Read the model definition and answer for the solid it produces. Units are mm, in the model's axes. Face numbers are marked on the shaded views. A direction names the side the tool comes from. Round coordinates to 2 decimals unless told otherwise and drop trailing zeros. Order: outer loops, then holes, each group sorted by start corner. A loop starts at its lowest first (then second) coordinate and runs counter-clockwise, first axis right, second up.
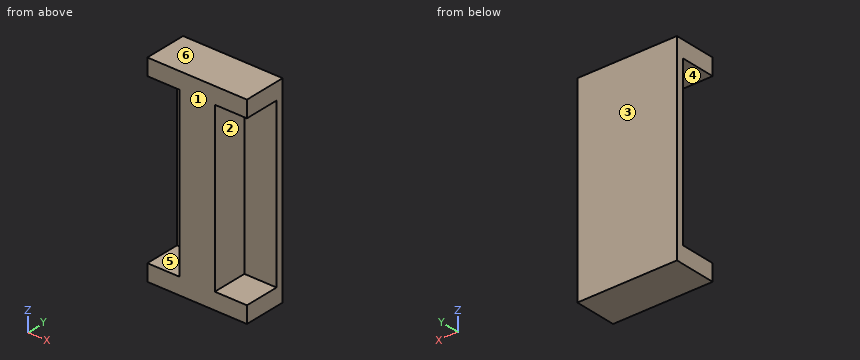
from build123d import *

# Parameters (mm, degrees)
F0_W     = 609.6
F0_H     = 1219.2
F1_DEPTH = 44.45
F2_W     = 609.6
F2_H     = 101.6
F3_DEPTH = 215.9
F4_W     = 215.9
F4_H     = 1016
F5_DEPTH = 260.35


with BuildPart() as f1:
    # F0 (on Front) → F1 (new body)
    with BuildSketch(Plane.XZ):
        Rectangle(F0_W, F0_H)
    extrude(amount=F1_DEPTH)

    # F2 (on face) → F3 (join)
    with BuildSketch(Plane.XZ.offset(44.45)):
        with Locations((0, 558.8)):
            Rectangle(F2_W, F2_H)
        with Locations((0, -558.8)):
            Rectangle(F2_W, F2_H)
    extrude(amount=F3_DEPTH)

    # F4 (on Front) → F5 (join)
    with BuildSketch(Plane.XZ):
        Rectangle(F4_W, F4_H)
    extrude(amount=F5_DEPTH)


solid = f1.part
Q1. For the marked faces 1 and 2, determine the directions among +Z, -Z, +X, -X, +Y, -Y from which every point of the face is accessible in a straight line to the end or side of a thin tool.
Outcome:
face 1: +Z, -Z, +X, -X, -Y
face 2: +X, -Y
Q2. A cutting plane is placed at B-B, the plane x = 126.5. Give the vertices of the cut face in (y, z), plus the area to 3 significant figures.
Outcome:
outline: (-260.35, -609.6) - (0, -609.6) - (0, 609.6) - (-260.35, 609.6) - (-260.35, 508) - (-44.45, 508) - (-44.45, -508) - (-260.35, -508) - close
area: 98,100 mm2
Q3. Flat-ended cylindrical pins translate along their axes: pin 1 (5 mm diameter, centred on y = -121, z = 459.5, fed in from +X); pin 2 (2 mm diameter, centred on y = -191, z = 345, fed in from -X); pin 3 (2 mm diameter, centred on x = -76, z = 45, fed in from +Y). Find the tip coordinate at first contact, or state that the pin passes through.
Outcome:
pin 1: stops at x = 107.95
pin 2: stops at x = -107.95
pin 3: stops at y = 0
Q4. Straight lines are drawn through the part: probe 1 along Z at (x, y) = (135.5, -141.5); probe 2 along Y at (x, z) = (157, -261.5); probe 3 along X at (y, z) = (-156, -88). For each, find the intervals that lie inside material, in ascending order.
Outcome:
probe 1: z = -609.6 to -508, 508 to 609.6
probe 2: y = -44.45 to 0
probe 3: x = -107.95 to 107.95
Q5. For a pull along Z with two mould halves and no side action, classify the marked faces 3, 4, 5 and 6 as released by +Z, released by -Z, zero draft, split by the parting line, or undercut.
Outcome:
face 3: zero draft
face 4: undercut
face 5: undercut
face 6: released by +Z
Q6. A cutting plane is placed at C-C, the plane z = 139. Give the vertices of the cut face in (x, y), plus the area to 3 significant figures.
Outcome:
outline: (-304.8, -44.45) - (-107.95, -44.45) - (-107.95, -260.35) - (107.95, -260.35) - (107.95, -44.45) - (304.8, -44.45) - (304.8, 0) - (-304.8, 0) - close
area: 73,700 mm2
Q7. A cutting plane is placed at A-A, the plane y = -208.5. Give the vertices of the cut face in (x, z).
Outcome:
outline: (-304.8, -609.6) - (304.8, -609.6) - (304.8, -508) - (107.95, -508) - (107.95, 508) - (304.8, 508) - (304.8, 609.6) - (-304.8, 609.6) - (-304.8, 508) - (-107.95, 508) - (-107.95, -508) - (-304.8, -508) - close
